Can you work these out from the model? Positions are in its coordinate system, mm. Give positions to 0.01 mm unless a question says otherwise; leave off trailing zeros. Write each loop counter-clockwise with the first axis right and the second up, starting at its lowest first coordinate (ties: lowest second). Pieces come first, ordered by that corner, then holes.
```python
from build123d import *

# Parameters (mm, degrees)
BOSS_EXTRUDE1_DEPTH = 2.54
SKETCH2_W           = 7.62
SKETCH2_H           = 7.62
BOSS_EXTRUDE2_DEPTH = 1.27


with BuildPart() as part:
    # Sketch1 → Boss-Extrude1 (new body)
    with BuildSketch(Plane(origin=(0, 0, 0), x_dir=(1, 0, 0), z_dir=(0, 1, 0))):
        Polygon((0, 0), (0, 101.6), (-101.6, 101.6), (-101.6, -50.8), (254, -50.8), (254, 0), align=None)
    extrude(amount=BOSS_EXTRUDE1_DEPTH)

    # Sketch2 → Boss-Extrude2 (add)
    with BuildSketch(Plane(origin=(0, 2.54, 0), x_dir=(1, 0, 0), z_dir=(0, 1, 0))):
        with Locations((-92.71, 92.71)):
            Rectangle(SKETCH2_W, SKETCH2_H)
        with Locations((-92.71, 85.09)):
            Rectangle(SKETCH2_W, SKETCH2_H)
        with Locations((-92.71, 77.47)):
            Rectangle(SKETCH2_W, SKETCH2_H)
    extrude(amount=BOSS_EXTRUDE2_DEPTH)


solid = part.part
```
1) Suppose I cut it at B-B on z = -87.5. Write out the boundary of the cut face in (x, y).
Values follow:
outline: (-101.6, 0) - (0, 0) - (0, 2.54) - (-88.9, 2.54) - (-88.9, 3.81) - (-96.52, 3.81) - (-96.52, 2.54) - (-101.6, 2.54) - close
2) Suppose I cut it at D-D on z = 23.5. Write out the boundary of the cut face in (x, y), plus the area to 3 significant figures.
Values follow:
outline: (-101.6, 0) - (254, 0) - (254, 2.54) - (-101.6, 2.54) - close
area: 903 mm2
3) Please list where these lines run through material, in increasing order: L1, parallel to X at y = 0.25, z = -45.5; L2, parallel to Z at x = 164, y = 1.05; L3, parallel to Y at x = -33.5, z = -17.5.
Values follow:
L1: x = -101.6 to 0
L2: z = 0 to 50.8
L3: y = 0 to 2.54
4) Suppose I cut it at C-C on x = -29. Write out the boundary of the cut face in (y, z), plus the area to 3 significant figures.
Values follow:
outline: (0, -101.6) - (2.54, -101.6) - (2.54, 50.8) - (0, 50.8) - close
area: 387 mm2
5) For pin 1 Ø1.4 at (y, z) = (3.5, -82) entering from +X; pin 2 Ø1.5 at (x, y) = (127.5, 2.5) entering from -Z; pin 3 Ø0.6 at (y, z) = (3, -85.5) entering from -X; pin 4 Ø1 at (x, y) = (-94, 3) entering from +Z, each with a flat end and sliding along its axis, tell me the tip position at first contact or that it passes through.
Values follow:
pin 1: stops at x = -88.9
pin 2: stops at z = 0
pin 3: stops at x = -96.52
pin 4: stops at z = 50.8
6) Suppose I cut it at A-A on y = 1.95. Write out the boundary of the cut face in (x, z), plus the area to 3 significant figures.
Values follow:
outline: (-101.6, -101.6) - (0, -101.6) - (0, 0) - (254, 0) - (254, 50.8) - (-101.6, 50.8) - close
area: 28,400 mm2
